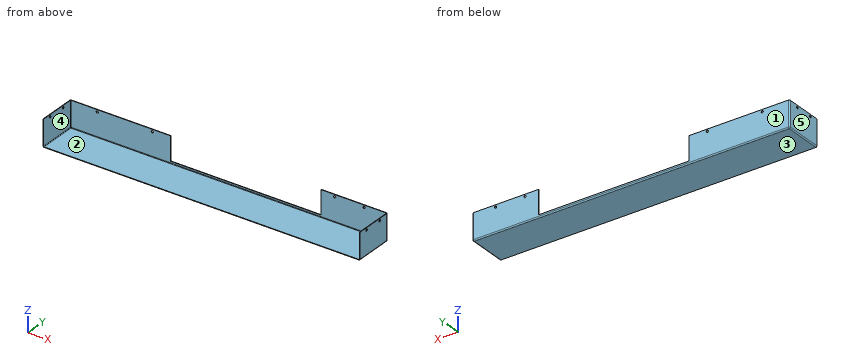
from build123d import *

# Parameters (mm, degrees)
SKETCH_1_W          = 864
SKETCH_1_H          = 105
EXTRUDE_1_DEPTH     = 72
FILLET_1_R          = 3
SHELL_1_T           = -1.5
SKETCH_3_W          = 410
SKETCH_3_H          = 65
CUT_EXTRUDE_2_DEPTH = 65
SKETCH_4_R          = 3
CUT_EXTRUDE_3_DEPTH = 874.329834599
SKETCH_5_R          = 3
CUT_EXTRUDE_4_DEPTH = 10


with BuildPart() as part:
    # 草图1 → 凸台-拉伸1 (new body)
    with BuildSketch(Plane.XY):
        with Locations((432, 52.5)):
            Rectangle(SKETCH_1_W, SKETCH_1_H)
    extrude(amount=EXTRUDE_1_DEPTH)

    # 圆角1
    fillet_1_edges = [part.edges().sort_by_distance(p)[0] for p in [
        (432, 105, 0),
        (864, 52.5, 0),
        (0, 52.5, 0),
        (0, 105, 36),
        (864, 105, 36),
    ]]
    fillet(fillet_1_edges, radius=FILLET_1_R)

    # 抽壳1
    shell_1_openings = [part.faces().sort_by_distance(p)[0] for p in [
        (432, 52.497793003, 72),
        (432, 0, 36.002193962),
    ]]
    offset(amount=SHELL_1_T, openings=shell_1_openings, kind=Kind.INTERSECTION)

    # 草图3 → 切除-拉伸2 (cut)
    with BuildSketch(Plane(origin=(0, 105, 0), x_dir=(1, 0, 0), z_dir=(0, 1, 0))):
        with Locations((479, -39.5)):
            Rectangle(SKETCH_3_W, SKETCH_3_H)
    extrude(amount=-CUT_EXTRUDE_2_DEPTH, mode=Mode.SUBTRACT)

    # 草图4 → 切除-拉伸3 (cut, through all)
    with BuildSketch(Plane(origin=(864, 0, 0), x_dir=(0, 0, -1), z_dir=(1, 0, 0))):
        with Locations((-66, 75)):
            Circle(SKETCH_4_R)
        with Locations((-66, 25)):
            Circle(SKETCH_4_R)
    extrude(amount=-CUT_EXTRUDE_3_DEPTH, mode=Mode.SUBTRACT)

    # 草图5 → 切除-拉伸4 (cut)
    with BuildSketch(Plane(origin=(0, 105, 0), x_dir=(1, 0, 0), z_dir=(0, 1, 0))):
        with Locations(Location((721, -66, 0), (0, 0, 270))):
            Circle(SKETCH_5_R)
        with Locations(Location((801, -66, 0), (0, 0, 270))):
            Circle(SKETCH_5_R)
        with Locations(Location((74, -66, 0), (0, 0, 270))):
            Circle(SKETCH_5_R)
        with Locations(Location((224, -66, 0), (0, 0, 270))):
            Circle(SKETCH_5_R)
    extrude(amount=-CUT_EXTRUDE_4_DEPTH, mode=Mode.SUBTRACT)


solid = part.part
The listing builds one solid part. Answer for the finished solid, in the listing's coordinates (mm). Face numbers are marked on the shaded views. A direction names the side the tool comes from. Round coordinates to 2 decimals unless told otherwise and drop trailing zeros. Loops run counter-clockwise (first coordinate to the right, second up) from the corner with the lowest first, then second, coordinate; pieces in that order, holes last. Notation, with made-up numbers: M 53,9 L 103,9 A12 cw 103,22 Z; hole C 50.5,-17.75 d9. An arc over 180 degrees is marked long. Return JSON: item names as keys, results as strings.
Q1. Find section C-C, the plane x = 236.5. Determine the outline of the cut face in (y, z).
Results list:
{"outline": "M 0,0 L 102,0 A3 ccw 105,3 L 105,72 L 103.5,72 L 103.5,3 A1.5 cw 102,1.5 L 0,1.5 Z"}
Q2. Each of these flat-tipped pins is pushed along its axis until it touches: pin 1 Ø5 at (x, z) = (251, 64.5) entering from -Y; pin 2 Ø1.2 at (x, y) = (533.5, 104) entering from +Z; pin 3 Ø2 at (x, y) = (255, 53.5) entering from +Z. Where does it stop, or does it pass through?
Results list:
{"pin 1": "stops at y = 103.5", "pin 2": "stops at z = 7", "pin 3": "stops at z = 1.5"}
Q3. Find section A-A, the plane x = 666.5. Determine the outline of the cut face in (y, z).
Results list:
{"outline": "M 0,0 L 102,0 A3 ccw 105,3 L 105,7 L 103.5,7 L 103.5,3 A1.5 cw 102,1.5 L 0,1.5 Z"}
Q4. The mould has two halves that part along X. Classify the marked faces 3, 4 and 5: released by +X, released by -X, zero draft, split by the parting line, or undercut.
Results list:
{"face 3": "zero draft", "face 4": "undercut", "face 5": "released by -X"}
Q5. Find section B-B, the plane y = 8. Determine the outline of the cut face in (x, z), plus the area to 3 significant figures.
Results list:
{"outline": "M 0,3 A3 ccw 3,0 L 861,0 A3 ccw 864,3 L 864,72 L 862.5,72 L 862.5,3 A1.5 cw 861,1.5 L 3,1.5 A1.5 cw 1.5,3 L 1.5,72 L 0,72 Z", "area": "1,500 mm2"}
Q6. Which of the six approach directions +Z, -Z, +X, -X, +Y, -Y give full straight-line access (tool end or side, diameter ignored) to the marked faces 1 and 2?
Results list:
{"face 1": "+Z, -Z, +X, -X, +Y", "face 2": "+Z, -Y"}
Q7. Find the intervals of material crossed by line 1 along X through (y, z) = (90.5, 36); line 2 along Y through (x, z) = (863, 66); line 3 along Y through (x, z) = (42, 19), in increasing order. Write a range as from..to.
Results list:
{"line 1": "x = 0..1.5, 862.5..864", "line 2": "y = 0..22, 28..72, 78..104.24", "line 3": "y = 103.5..105"}
